Geometry: final body of the model. Coordinates: model frame, mm. Face numbers are marked on the shaded views. Round coordinates to 2 decimals unless told otherwise and drop trailing zeros. Loops run counter-clockwise (first coordinate to the right, second up) from the corner with the lowest first, then second, coordinate; pieces in that order, holes last. Notation, with made-up numbers: (-31.75, 6) - (-18.75, 6) arc R24 cw to (-18.75, 37) - close; hole circle Ø9 at (17, 71.5). An arc over 180 degrees is marked (long way). Use CSV: the item, a comma, the result in double quotes.
from build123d import *

# Parameters (mm, degrees)
CROQUIS2_R              = 1.95
SALIENTE_EXTRUIR1_DEPTH = 8
C_PULA1_FACE_RADIUS     = 1.95
C_PULA1_HEIGHT          = 5.3
CROQUIS11_W             = 9.35
CROQUIS11_H             = 20
SALIENTE_EXTRUIR3_DEPTH = 2
FILLET1_R               = 1
FILLET2_R               = 1
FILLET3_R               = 3


with BuildPart() as part:
    # Croquis2 → Saliente-Extruir1 (new body)
    with BuildSketch(Plane(origin=(0, 0, 0), x_dir=(1, 0, 0), z_dir=(0, 1, 0))):
        with Locations(Location((0, 0, 0), (0, 0, 270))):
            Circle(CROQUIS2_R)
    extrude(amount=SALIENTE_EXTRUIR1_DEPTH)

    # Cúpula1: a dome of height H over a round flat face of radius A is a cap of a sphere of radius (A * A + H * H) / (2 * H)
    c_pula1_r = (C_PULA1_FACE_RADIUS * C_PULA1_FACE_RADIUS + C_PULA1_HEIGHT * C_PULA1_HEIGHT) / (2 * C_PULA1_HEIGHT)
    c_pula1_base = Plane((0, 8, 0), z_dir=(0, 1, 0))
    with Locations(c_pula1_base.offset(C_PULA1_HEIGHT - c_pula1_r)):
        c_pula1_ball = Sphere(c_pula1_r, mode=Mode.PRIVATE)
    add(split(c_pula1_ball, bisect_by=c_pula1_base, keep=Keep.TOP, mode=Mode.PRIVATE))

    # Croquis11 → Saliente-Extruir3 (add)
    with BuildSketch(Plane(origin=(0, 0, 0), x_dir=(-1, 0, 0), z_dir=(0, -1, 0))):
        Rectangle(CROQUIS11_W, CROQUIS11_H)
    extrude(amount=SALIENTE_EXTRUIR3_DEPTH)

    # Fillet1
    fillet1_edges = [part.edges().sort_by_distance(p)[0] for p in [
        (0, 0, -1.95),
        (0, 0, -10),
        (4.675, 0, 0),
        (-4.675, 0, 0),
        (0, 0, 10),
    ]]
    fillet(fillet1_edges, radius=FILLET1_R)

    # Fillet2
    # the kernel refuses this fillet: 1 mm, written as the material it takes off along each edge
    with BuildSketch(Plane(origin=(-3.675, -1, 9), x_dir=(0, 0, 1), z_dir=(-1, 0, 0))) as fillet2_piece_1_section:
        Polygon((0, 0), (FILLET2_R, 0), (FILLET2_R, FILLET2_R), (0, FILLET2_R), align=None)
    fillet2_piece_1 = extrude(amount=FILLET2_R, mode=Mode.PRIVATE)
    fillet2_piece_1 = fillet2_piece_1 - Plane(origin=(-3.675, -1, 9), x_dir=(0, -0.7071067811865475, -0.7071067811865475), z_dir=(-1, 0, 0)) * Sphere(FILLET2_R, mode=Mode.PRIVATE)
    add(fillet2_piece_1, mode=Mode.SUBTRACT)
    with BuildSketch(Plane(origin=(-3.675, -1, -9), x_dir=(-1, 0, 0), z_dir=(0, 0, -1))) as fillet2_piece_2_section:
        Polygon((0, 0), (FILLET2_R, 0), (FILLET2_R, FILLET2_R), (0, FILLET2_R), align=None)
    fillet2_piece_2 = extrude(amount=FILLET2_R, mode=Mode.PRIVATE)
    fillet2_piece_2 = fillet2_piece_2 - Plane(origin=(-3.675, -1, -9), x_dir=(0.7071067811865475, -0.7071067811865475, 0), z_dir=(0, 0, -1)) * Sphere(FILLET2_R, mode=Mode.PRIVATE)
    add(fillet2_piece_2, mode=Mode.SUBTRACT)
    with BuildSketch(Plane(origin=(3.675, -1, -9), x_dir=(1, 0, 0), z_dir=(0, 0, -1))) as fillet2_piece_3_section:
        Polygon((0, 0), (FILLET2_R, 0), (FILLET2_R, -FILLET2_R), (0, -FILLET2_R), align=None)
    fillet2_piece_3 = extrude(amount=FILLET2_R, mode=Mode.PRIVATE)
    fillet2_piece_3 = fillet2_piece_3 - Plane(origin=(3.675, -1, -9), x_dir=(-0.7071067811865475, -0.7071067811865475, 0), z_dir=(0, 0, -1)) * Sphere(FILLET2_R, mode=Mode.PRIVATE)
    add(fillet2_piece_3, mode=Mode.SUBTRACT)
    with BuildSketch(Plane(origin=(-4.675, -1, 10), x_dir=(0, 0, -1), z_dir=(0, -1, 0)), Plane(origin=(-4.675, -1, -10), x_dir=(1, 0, 0), z_dir=(0, -1, 0))) as fillet2_piece_4:
        with BuildLine():
            CenterArc((FILLET2_R, FILLET2_R), FILLET2_R, 180, 90)
            Line((0, FILLET2_R), (0, 0))
            Line((0, 0), (FILLET2_R, 0))
        make_face()
    extrude(amount=3.5, mode=Mode.SUBTRACT)
    with BuildSketch(Plane(origin=(4.675, -1, -10), x_dir=(-1, 0, 0), z_dir=(0, -1, 0))) as fillet2_piece_5:
        with BuildLine():
            CenterArc((FILLET2_R, -FILLET2_R), FILLET2_R, 90, 90)
            Line((0, -FILLET2_R), (0, 0))
            Line((0, 0), (FILLET2_R, 0))
        make_face()
    extrude(amount=3.5, mode=Mode.SUBTRACT)

    # Fillet3
    fillet3_edges = [part.edges().sort_by_distance(p)[0] for p in [
        (0, 8, -1.95),
    ]]
    fillet(fillet3_edges, radius=FILLET3_R)


solid = part.part
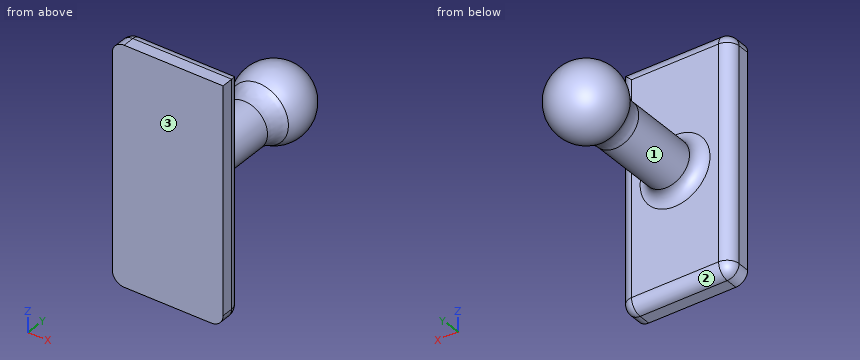
Item 1: Material intervals for line 1 (Y direction, x = 3.75, z = -6.25); line 2 (Y direction, x = 2.25, z = 0); line 3 (Y direction, x = 0.25, z = 2.5), sorted ascending.
Final values:
line 1,"y = -2 to 0"
line 2,"y = -2 to 0.29, 8.19 to 12.29"
line 3,"y = -2 to 0.1, 8.64 to 11.95"
Item 2: Section B-B on z = 4.5. Return the cut outline in (x, y) (3 decimals), plus the area to 3 significant figures.
Final values:
outline,"(-4.675, -2) - (4.675, -2) - (4.675, -1) arc R1 ccw to (3.675, 0) - (-3.675, 0) arc R1 ccw to (-4.675, -1) - close"
area,"18.3 mm²"
Item 3: Section C-C on y = -0.5. Return the cut outline in (x, z) (3 decimals), plus the area to 3 significant figures.
Final values:
outline,"(-4.541, -9) arc R0.866 ccw to (-3.675, -9.866) - (3.675, -9.866) arc R0.866 ccw to (4.541, -9) - (4.541, 9.866) - (-3.675, 9.866) arc R0.866 ccw to (-4.541, 9) - close"
area,"179 mm²"
Item 4: Pin query (flat end, axial travel): P1, Ø4, axis at x = -3.5, y = 5.5, coming from the +Z side; P2, Ø1.5, axis at x = 2, y = 5.5, coming from the +Z side; P3, Ø8, axis at y = 6, z = 1.5, coming from the +X side. Return the tip coordinate at first contact, or that it passes through.
Final values:
P1,"stops at z = 1.25"
P2,"stops at z = 1.5"
P3,"stops at x = 2.96"
Item 5: Section A-A on x = -3.25. Return the cut outline in (y, z).
Final values:
outline,"(-2, -10) - (-1, -10) arc R1 ccw to (0, -9) - (0, 9) arc R1 ccw to (-1, 10) - (-2, 10) - close"
Item 6: Mould query, pull axis Y, two halves, no side actions, for the marked faces 1, 2 and 3. Classes: released by +Y, released by -Y, zero draft, split by the parting line, or undercut.
Final values:
face 1,"undercut"
face 2,"released by +Y"
face 3,"released by -Y"
Item 7: Section D-D on y = 12. Return the cut outline in (x, z), plus the area to 3 significant figures.
Final values:
outline,"circle Ø4.95 at (0, 0)"
area,"19.3 mm²"
